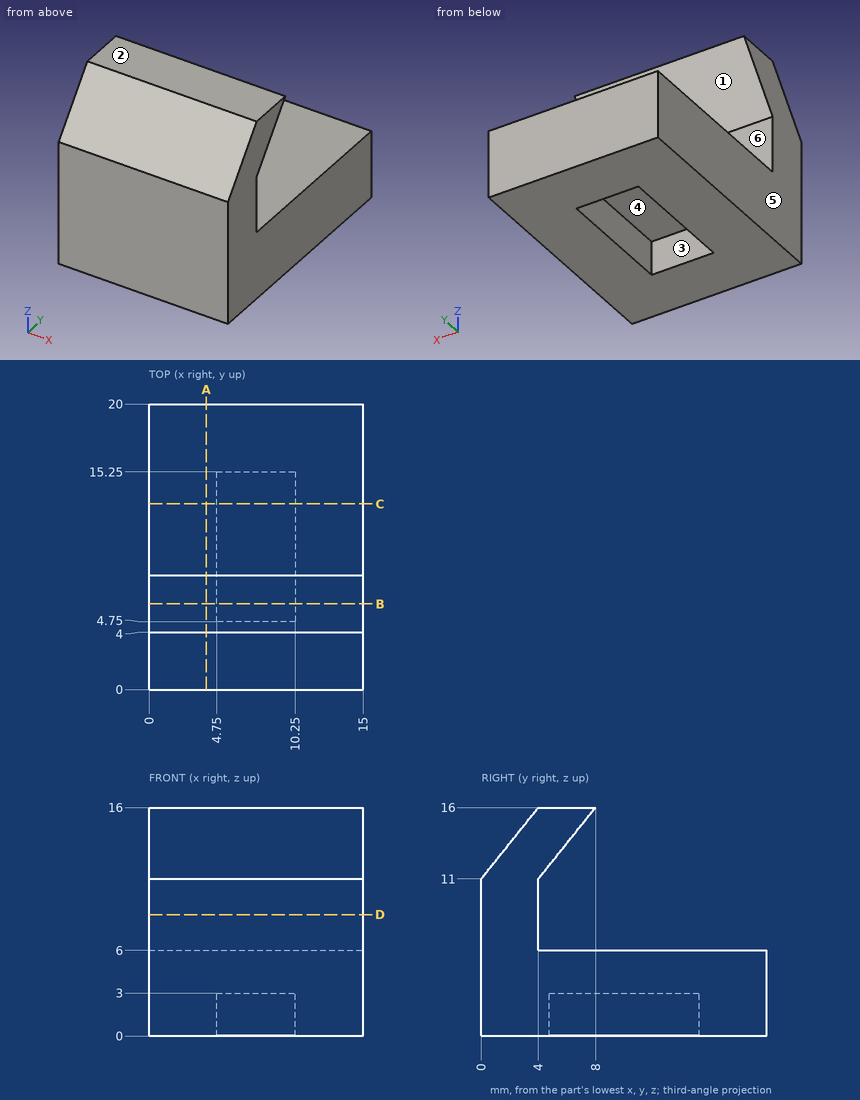
Geometry: see drawing. Coordinates: mm, zero at the bounding-box minimum. A direction names the side the tool comes from. Round coordinates to 2 decimals unless told otherwise and drop trailing zeros. Loops run counter-clockwise (first coordinate to the right, second up) from the corner with the lowest first, then second, coordinate; pieces in that order, holes last. Notation, with made-up numbers: M -38,44 L 0,44 A20 cw 0,71 Z; hole C -31.75,8 d11. An arc over 180 degrees is marked long. Use a Markdown table: item, result. Add a question column.
1. Reachability of the marked faces 1, 2 and 3 from +Z, -Z, +X, -X, +Y, -Y: full face, straight path, thin tool, end or side. Return the list, or none.
2. Line query: line 1 (X direction, y = 8, z = 1.5); line 2 (Y direction, x = 8.5, z = 1.25); line 3 (Y direction, x = 9.5, z = 7.75). Output: solid intervals per line, ascending.
3. Section query D-D on z = 8.5. Return the cut outline in (x, y).
4. Contact query for flat-ended pins moving along their axis: P1, Ø6, axis at x = 5.5, y = 13, coming from the -Z side; P2, Ø1, axis at x = 1.5, y = 16.5, coming from the +Z side; P3, Ø3, axis at x = 4.5, z = 8, coming from the +Y side. Output: stop coordinate, or through.
5. Mould query, pull axis Y, two halves, no side actions, for the marked faces 4, 5 and 6. Classes: pulls with the +Y half, pulls with the -Y half, needs draft (parallel to the pull), parting line crosses it, or undercut.
6. Section query A-A on x = 4. Return the cut outline in (y, z).
7. Section query B-B on y = 6. Return the cut outline in (x, z).
8. Section query C-C on y = 13. Return the cut outline in (x, z), then the cut area to 3 significant figures.
Reported:
| question | item | result |
|---|---|---|
| 1 | face 1 | +X, -X, +Y |
| 1 | face 2 | +Z, +X, -X, +Y, -Y |
| 1 | face 3 | -Z |
| 2 | line 1 | x = 0 to 4.75, 10.25 to 15 |
| 2 | line 2 | y = 0 to 4.75, 15.25 to 20 |
| 2 | line 3 | y = 0 to 4 |
| 3 | outline | M 0,0 L 15,0 L 15,4 L 0,4 Z |
| 4 | P1 | stops at z = 0 |
| 4 | P2 | stops at z = 6 |
| 4 | P3 | stops at y = 4 |
| 5 | face 4 | undercut |
| 5 | face 5 | needs draft |
| 5 | face 6 | pulls with the +Y half |
| 6 | outline | M 0,0 L 20,0 L 20,6 L 4,6 L 4,11 L 8,16 L 4,16 L 0,11 Z |
| 7 | outline | M 0,0 L 4.75,0 L 4.75,3 L 10.25,3 L 10.25,0 L 15,0 L 15,6 L 0,6 Z; M 0,13.5 L 15,13.5 L 15,16 L 0,16 Z |
| 8 | outline | M 0,0 L 4.75,0 L 4.75,3 L 10.25,3 L 10.25,0 L 15,0 L 15,6 L 0,6 Z |
| 8 | area | 73.5 mm² |
